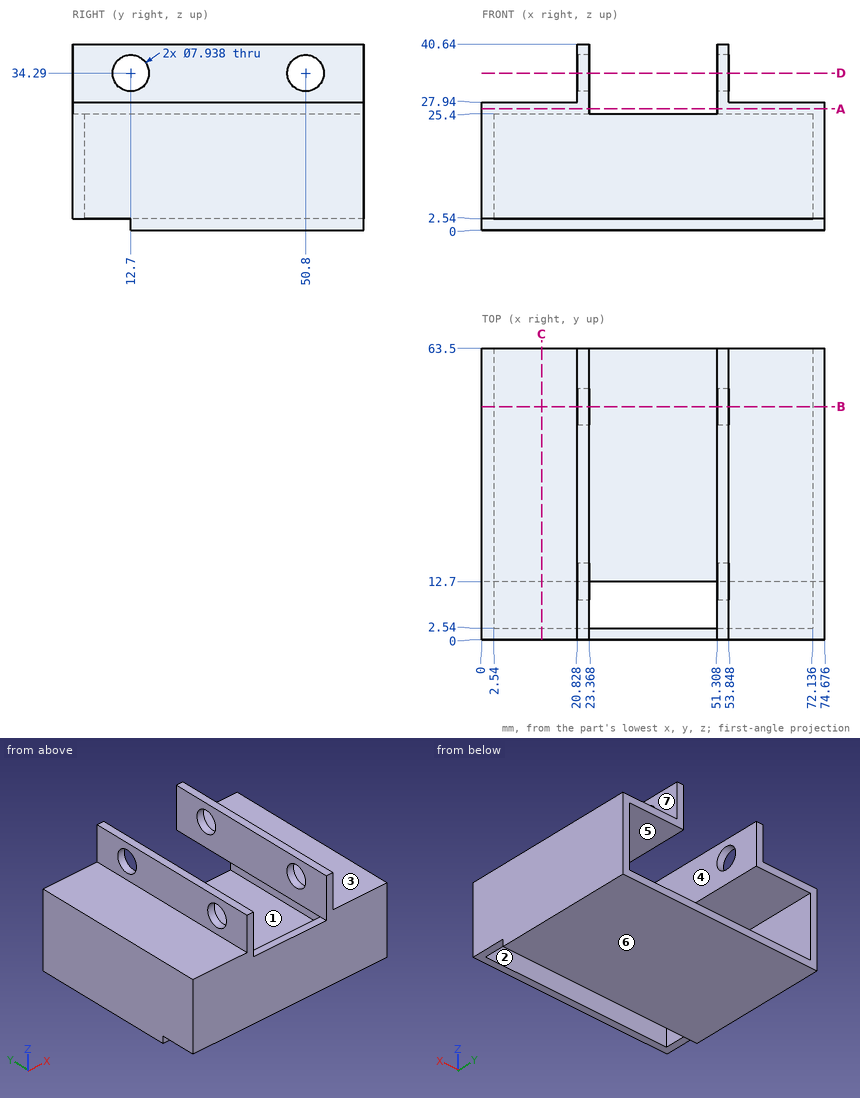
Part print with two shaded views. Sizes in mm from the minimum x, y, z corner. A direction names the side the tool comes from. Give positions to 0.01 mm unless a question says otherwise; leave off trailing zeros. Order: outer loops, then holes, each group sorted by start corner. A loop starts at its lowest first (then second) coordinate and runs counter-clockwise, first axis right, second up. Notation, with made-up numbers: M 71,-31.5 L 114,-31.5 A18 ccw 114,-4.5 Z; hole C -35.5,26 d4. An arc over 180 degrees is marked long. Write item = value, one per line.
Q1. Cut at A-A, the plane z = 26.5. List the corners of the cut face in (x, y) (1 decimal).
Derived:
outline = M 0,0 L 23.4,0 L 23.4,63.5 L 0,63.5 Z; M 51.3,0 L 74.7,0 L 74.7,63.5 L 51.3,63.5 Z
Q2. Tool access for the marked faces 1, 2, 3 and 4: list every direction of +Z, -Z, +X, -X, +Y, -Y with a clear straight run to the whole face (end or side of a thin tool).
Derived:
face_1 = +Y
face_2 = -Z, +Y
face_3 = +Z, +X, +Y, -Y
face_4 = +Z, +Y, -Y
Q3. Drill centre lines: line 1 (Y direction, x = 21, z = 34); line 2 (Z direction, x = 52.2, y = 50.8); line 3 (X direction, y = 60, z = 22) (1 decimal). Where is each one in solid material? Low to high. Write a range as [from, to].
Derived:
line_1 = [0, 8.74], [16.66, 46.84], [54.76, 63.5]
line_2 = [0, 2.54], [25.4, 30.32], [38.26, 40.64]
line_3 = [0, 2.5], [72.1, 74.7]
Q4. Two-plate mould, pull along X, no slides. Class the marked faces 5, 6 and 7: pulls with the +X half, pulls with the -X half, needs draft (parallel to the pull), parting line crosses it, or undercut.
Derived:
face_5 = undercut
face_6 = needs draft
face_7 = pulls with the +X half
Q5. Cut at D-D, the plane z = 34.29. List the corners of the cut face in (x, y), then the cut area to 3 significant figures.
Derived:
outline = M 20.83,0 L 23.37,0 L 23.37,8.73 L 20.83,8.73 Z; M 20.83,16.67 L 23.37,16.67 L 23.37,46.83 L 20.83,46.83 Z; M 20.83,54.77 L 23.37,54.77 L 23.37,63.5 L 20.83,63.5 Z; M 51.31,0 L 53.85,0 L 53.85,8.73 L 51.31,8.73 Z; M 51.31,16.67 L 53.85,16.67 L 53.85,46.83 L 51.31,46.83 Z; M 51.31,54.77 L 53.85,54.77 L 53.85,63.5 L 51.31,63.5 Z
area = 242 mm2
Q6. Cut at B-B, the plane y = 50.8. List the corners of the cut face in (x, z) (1 decimal).
Derived:
outline = M 0,0 L 74.7,0 L 74.7,27.9 L 53.8,27.9 L 53.8,30.3 L 51.3,30.3 L 51.3,25.4 L 72.1,25.4 L 72.1,2.5 L 2.5,2.5 L 2.5,25.4 L 23.4,25.4 L 23.4,30.3 L 20.8,30.3 L 20.8,27.9 L 0,27.9 Z; M 20.8,38.3 L 23.4,38.3 L 23.4,40.6 L 20.8,40.6 Z; M 51.3,38.3 L 53.8,38.3 L 53.8,40.6 L 51.3,40.6 Z
Q7. Flat gauge pins, fed straight in: pin 1 (1 mm diameter, centred on y = 7.5, z = 28.5, fed in from -X); pin 2 (0.8 mm diameter, centred on x = 44.5, z = 1, fed in from -Y); pin 3 (10.5 mm diameter, centred on y = 12.7, z = 34.29, fed in from +X). Where does each tip first touch, or does it go through?
Derived:
pin_1 = 20.83
pin_2 = 12.7
pin_3 = 53.85
Q8. Cut at C-C, the plane x = 13. List the corners of the cut face in (y, z).
Derived:
outline = M 0,2.54 L 2.54,2.54 L 2.54,25.4 L 63.5,25.4 L 63.5,27.94 L 0,27.94 Z; M 12.7,0 L 63.5,0 L 63.5,2.54 L 12.7,2.54 Z
